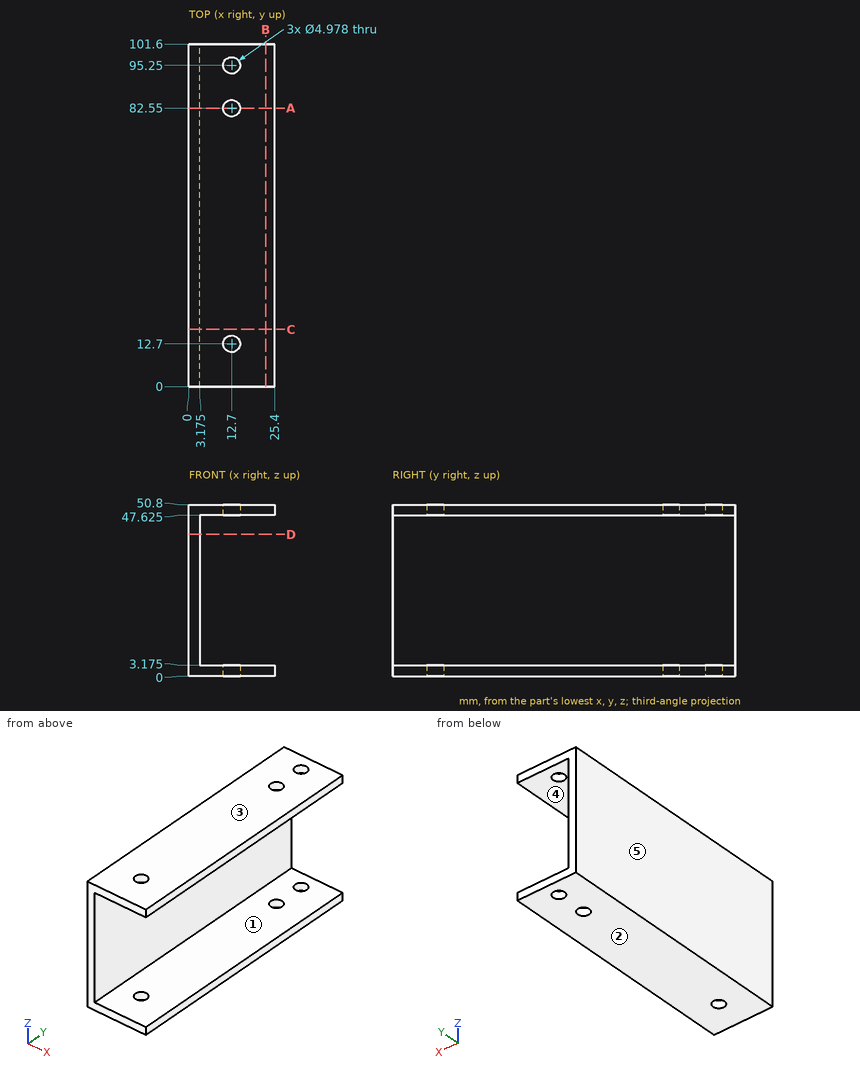
Drawing for the job (mm, zero at the part's lowest x, y, z). A direction names the side the tool comes from. Give positions to 0.01 mm unless a question says otherwise; leave off trailing zeros. Write each loop counter-clockwise with the first axis right and the second up, starting at its lowest first coordinate (ties: lowest second). Pieces come first, ordered by that corner, then holes. Notation, with made-up numbers: M 79,48.5 L 110,48.5 A21 cw 110,74.5 Z; hole C 3,-5.5 d7. An arc over 180 degrees is marked long. Return JSON: item names as keys, results as strings. Group by question number.
(1) Band-saw the part on C-C (y = 17). Give the cut face in (x, z) (1 decimal).
(2) Drill centre lines: L1, parallel to Y at x = 12.7, z = 48.85; L2, parallel to Z at x = 19.5, y = 73.5 (1 decimal); L3, parallel to X at y = 95, z = 2. Where is each one in solid material? Low to high. Write a range as [from, to].
(3) Mould opens along Z. For the marked faces 3, 4 and 5 say: pulls with the +Z half, pulls with the -Z half, needs draft (parallel to the pull), parting line crosses it, or undercut.
(4) Flat gauge pins, fed straight in: pin 1 Ø12 at (y, z) = (91, 14) entering from +X (3 decimals); pin 2 Ø3 at (x, y) = (12.7, 12.7) entering from -Z. Where does each tip first touch, or does it go through?
(5) Band-saw the part on D-D (z = 42). Give the cut face in (x, y) (1 decimal).
(6) Band-saw the part on B-B (x = 22.75). Give the cut face in (y, z) (1 decimal), and give its area (3 significant figures).
(7) Band-saw the part on A-A (y = 82.55). Give the cut face in (x, z) (1 decimal), and give its area (3 significant figures).
(8) 3-axis set-ups, long thin cutter, end or side, ignore diameter. For the marked faces 1 and 2: which of +Z, -Z, +X, -X, +Y, -Y reach the whole face in a straight line?
Entries:
{
 "1": {"outline": "M 0,0 L 25.4,0 L 25.4,3.2 L 3.2,3.2 L 3.2,47.6 L 25.4,47.6 L 25.4,50.8 L 0,50.8 Z"},
 "2": {"L1": "y = [0, 10.21], [15.19, 80.06], [85.04, 92.76], [97.74, 101.6]", "L2": "z = [0, 3.2], [47.6, 50.8]", "L3": "x = [0, 10.22], [15.18, 25.4]"},
 "3": {"face 3": "pulls with the +Z half", "face 4": "undercut", "face 5": "needs draft"},
 "4": {"pin 1": "stops at x = 3.175", "pin 2": "passes through"},
 "5": {"outline": "M 0,0 L 3.2,0 L 3.2,101.6 L 0,101.6 Z"},
 "6": {"outline": "M 0,0 L 101.6,0 L 101.6,3.2 L 0,3.2 Z; M 0,47.6 L 101.6,47.6 L 101.6,50.8 L 0,50.8 Z", "area": "645 mm^2"},
 "7": {"outline": "M 0,0 L 10.2,0 L 10.2,3.2 L 3.2,3.2 L 3.2,47.6 L 10.2,47.6 L 10.2,50.8 L 0,50.8 Z; M 15.2,0 L 25.4,0 L 25.4,3.2 L 15.2,3.2 Z; M 15.2,47.6 L 25.4,47.6 L 25.4,50.8 L 15.2,50.8 Z", "area": "271 mm^2"},
 "8": {"face 1": "+X, +Y, -Y", "face 2": "-Z, +X, -X, +Y, -Y"}
}
